Can you work these out from the drawing? Everything is in mm from the part's minimum corner. A direction names the side the tool comes from. Round coordinates to 2 decimals unless told otherwise and drop trailing zeros. Order: outer loops, then holes, each group sorted by start corner. A loop starts at its lowest first (then second) coordinate and runs counter-clockwise, first axis right, second up. Notation, with made-up numbers: M 78.5,65 L 89.5,65 A8 cw 89.5,79 Z; hole C 9.25,44 d3. An arc over 180 degrees is marked long. Write item = value, one per line. Start each with the question number.
Item 1: I want a section at C-C, the plane z = 1.75. State how many separate pieces and enclosed holes the cut face has, plus the area to 3 significant figures.
Item 2: Please list where these lines run through material, in increasing order: L1, parallel to X at y = 37, z = 3.75; L2, parallel to Z at x = 8.5, y = 28; L3, parallel to Y at x = 17, z = 7.75.
Item 3: I'm going to push a flat-ended pin straight in: P1, Ø12, axis at x = 21, y = 9, coming from the +Z side. Where does the tip first touch, or does it pass through?
Item 4: For the marked faces 1, 2, 3 and 4, which set-ups out of +Z, -Z, +X, -X, +Y, -Y let a thin tool reach every point of the face, with its end or its side?
Item 5: I want a section at D-D, the plane z = 10.25. List the corners of the cut face in (x, y) for me.
Item 6: I want a section at B-B, the plane x = 15.25. List the corners of the cut face in (y, z) for me, plus the area to 3 significant figures.
Item 7: I want a section at A-A, the plane y = 42.5. List the corners of the cut face in (x, z) for me.
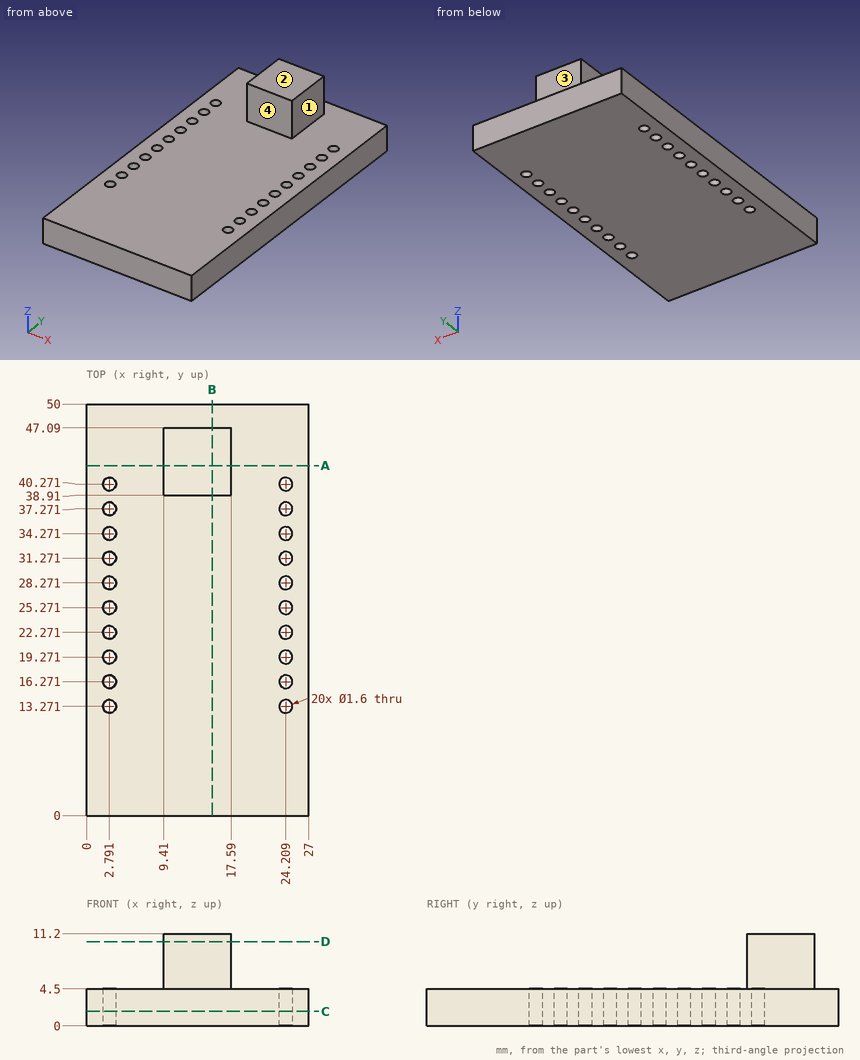
Filled in:
q1.separate_pieces = 1
q1.enclosed_holes = 20
q1.area = 1,310 mm^2
q2.L1 = 0 to 2.04, 3.54 to 23.46, 24.96 to 27
q2.L2 = 0 to 4.5
q2.L3 = 38.91 to 47.09
q3.P1 = 4.5
q4.face_1 = +Z, +X, +Y, -Y
q4.face_2 = +Z, +X, -X, +Y, -Y
q4.face_3 = +Z, +X, -X, +Y
q4.face_4 = +Z, +X, -X, -Y
q5.outline = M 9.41,38.91 L 17.59,38.91 L 17.59,47.09 L 9.41,47.09 Z
q6.outline = M 0,0 L 50,0 L 50,4.5 L 47.09,4.5 L 47.09,11.2 L 38.91,11.2 L 38.91,4.5 L 0,4.5 Z
q6.area = 280 mm^2
q7.outline = M 0,0 L 27,0 L 27,4.5 L 17.59,4.5 L 17.59,11.2 L 9.41,11.2 L 9.41,4.5 L 0,4.5 Z
